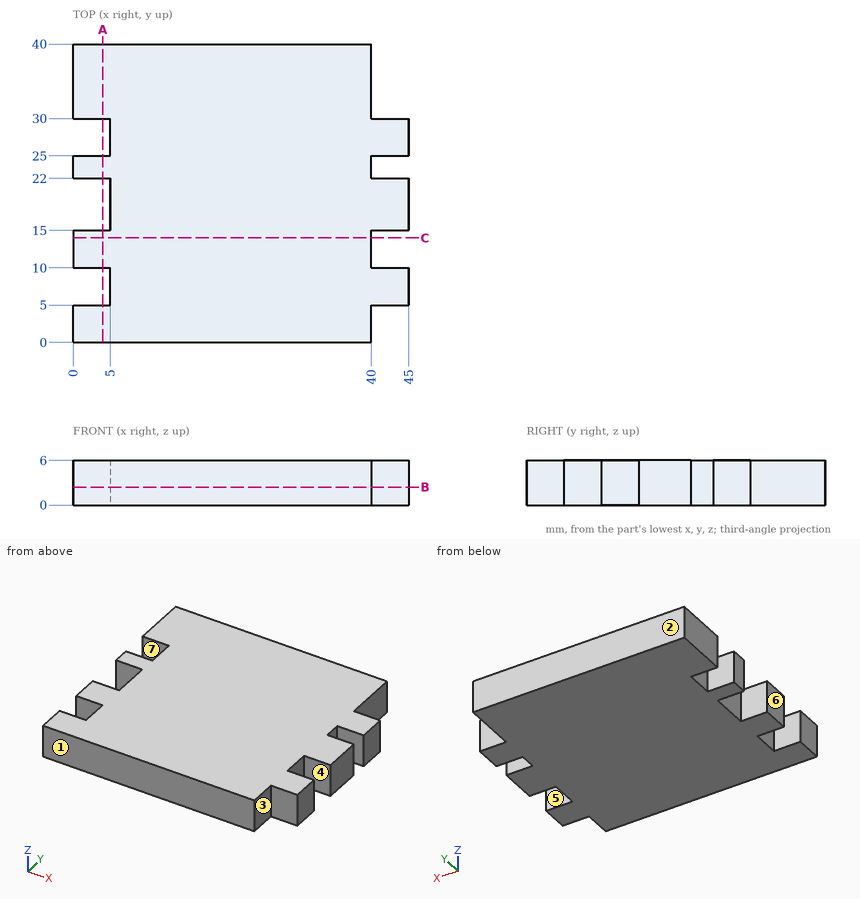
Geometry: see drawing. Coordinates: mm, zero at the bounding-box minimum. A direction names the side the tool comes from. Coordinates: 2 decimals unless noted, no trailing zeros. Write each loop counter-clockwise with the first axis right and the second up, starting at its lowest first coordinate (ties: lowest second). Pieces come first, ordered by that corner, then holes. Notation, with made-up numbers: M 47,66 L 98,66 A7 cw 98,74 Z; hole C 30.25,-15.5 d4. An arc over 180 degrees is marked long. Use CSV: the item, a comma, the result in double quotes. Start each with the question number.
1. Cut plane B-B on z = 2.4. Return the cut outline in (x, y), plus the area to 3 significant figures.
2. First-contact query: P1, Ø2.5, axis at x = 43.5, z = 2.5, coming from the -Y side; P2, Ø1.8, axis at y = 18, z = 3.5, coming from the -X side; P3, Ø1.5, axis at y = 12.5, z = 2.5, coming from the +X side. Flat tips, straight axial feed; report the tip coordinate or a pass-through.
3. Cut plane C-C on y = 14. Return the cut outline in (x, z).
4. Reachability of the marked faces 5, 6 and 7 from +Z, -Z, +X, -X, +Y, -Y: full face, straight path, thin tool, end or side. Return the list, or none.
5. Cut plane A-A on x = 4. Return the cut outline in (y, z), plus the area to 3 significant figures.
6. Mould query, pull axis Y, two halves, no side actions, for the marked faces 1, 2, 3 and 4. Classes: pulls with the +Y half, pulls with the -Y half, needs draft (parallel to the pull), parting line crosses it, or undercut.
7. Ray query, probe 1 along Y at (x, z) = (40.5, 4.15); probe 2 along Y at (x, z) = (3.5, 0.3); probe 3 along X at (y, z) = (7, 5). Return the intervals inside material, ascending.
Entries:
1,outline,"M 0,0 L 40,0 L 40,5 L 45,5 L 45,10 L 40,10 L 40,15 L 45,15 L 45,22 L 40,22 L 40,25 L 45,25 L 45,30 L 40,30 L 40,40 L 0,40 L 0,30 L 5,30 L 5,25 L 0,25 L 0,22 L 5,22 L 5,15 L 0,15 L 0,10 L 5,10 L 5,5 L 0,5 Z"
1,area,"1,600 mm²"
2,P1,"y = 5"
2,P2,"x = 5"
2,P3,"x = 40"
3,outline,"M 0,0 L 40,0 L 40,6 L 0,6 Z"
4,face 5,"+Z, -Z, +X"
4,face 6,"+Z, -Z, -X, +Y, -Y"
4,face 7,"+Z, -Z, -X"
5,outline,"M 0,0 L 5,0 L 5,6 L 0,6 Z; M 10,0 L 15,0 L 15,6 L 10,6 Z; M 22,0 L 25,0 L 25,6 L 22,6 Z; M 30,0 L 40,0 L 40,6 L 30,6 Z"
5,area,"138 mm²"
6,face 1,"pulls with the -Y half"
6,face 2,"pulls with the +Y half"
6,face 3,"needs draft"
6,face 4,"undercut"
7,probe 1,"5 to 10, 15 to 22, 25 to 30"
7,probe 2,"0 to 5, 10 to 15, 22 to 25, 30 to 40"
7,probe 3,"5 to 45"
